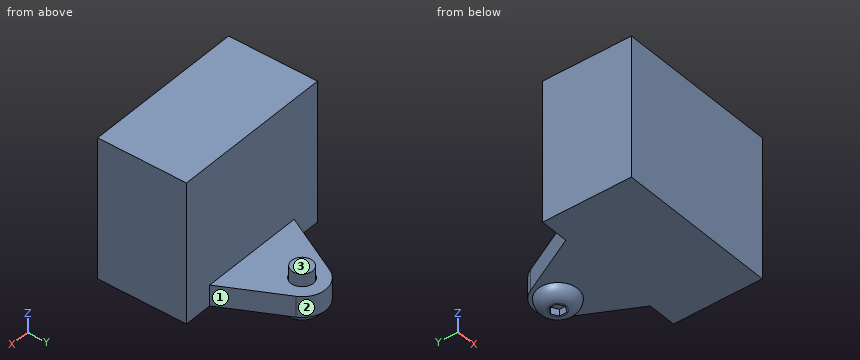
```python
from build123d import *

# Parameters (mm, degrees)
BOSS_EXTRUDE1_DEPTH = 4
SKETCH2_W           = 31
SKETCH2_H           = 17
BOSS_EXTRUDE2_DEPTH = 27
SKETCH4_R           = 2.15
CUT_EXTRUDE1_DEPTH  = 39.429285708
CUT_EXTRUDE2_DEPTH  = 1.3


with BuildPart() as part:
    # Sketch1 → Boss-Extrude1 (new body)
    with BuildSketch(Plane.XY.offset(-4)):
        with BuildLine():
            Line((-10, -9.6), (10, -9.6))
            Line((10, -9.6), (4.001428187, 2.058779362))
            ThreePointArc((4.001428187, 2.058779362), (0, 4.5), (-4.001428187, 2.058779362))
            Line((-4.001428187, 2.058779362), (-10, -9.6))
        make_face()
    extrude(amount=BOSS_EXTRUDE1_DEPTH)

    # Sketch2 → Boss-Extrude2 (add)
    with BuildSketch(Plane.XY.offset(-4)):
        with Locations((0, -18.1)):
            Rectangle(SKETCH2_W, SKETCH2_H)
    extrude(amount=BOSS_EXTRUDE2_DEPTH)

    # Sketch4 → Cut-Extrude1 (cut, through all)
    with BuildSketch(Plane.XY):
        Circle(SKETCH4_R)
    extrude(amount=-CUT_EXTRUDE1_DEPTH, mode=Mode.SUBTRACT)

    # Sketch5 → Revolve1 (revolve)
    with BuildSketch(Plane(origin=(0, 0, 0), x_dir=(0, 0, -1), z_dir=(1, 0, 0)), mode=Mode.PRIVATE) as revolve1_sk:
        with BuildLine():
            Line((-2.3, 0), (6.2, 0))
            Line((6.2, 0), (6.2, 1.6))
            ThreePointArc((6.2, 1.6), (5.555634919, 3.155634919), (4, 3.8))
            Line((4, 3.8), (4, 2))
            Line((4, 2), (-2.3, 2))
            Line((-2.3, 2), (-2.3, 0))
        make_face()
    revolve(revolve1_sk.sketch.rotate(Axis((0, 0, 2.3), (0, 0, -1)), 90), axis=Axis((0, 0, 2.3), (0, 0, -1)))

    # Sketch6 → Cut-Extrude2 (cut)
    with BuildSketch(Plane.XY.offset(-6.2)):
        Polygon((0, 1.443375673), (-1.25, 0.721687836), (-1.25, -0.721687836), (0, -1.443375673), (1.25, -0.721687836), (1.25, 0.721687836), align=None)
    extrude(amount=CUT_EXTRUDE2_DEPTH, mode=Mode.SUBTRACT)


solid = part.part
```
Work out the finished part from the listing and answer in its coordinate system (mm). Face numbers are marked on the shaded views. Give positions to 0.01 mm unless a question says otherwise; leave off trailing zeros. Order: outer loops, then holes, each group sorted by start corner. A loop starts at its lowest first (then second) coordinate and runs counter-clockwise, first axis right, second up. Notation, with made-up numbers: (42, -7.75) -> (72, -7.75) arc R24 cw to (72, 5.25) -> close; hole circle Ø3 at (51.25, 47). An arc over 180 degrees is marked (long way). Answer as CSV lines item,"result". Start each with the question number.
(1) Section B-B, the plane z = 9 is taken. Write down the section's boundary in (x, y), plus the area to 3 significant figures.
(2) Section C-C, the plane x = -5 is taken. Write down the section's boundary in (y, z).
(3) Section D-D, the plane y = -12.5 is taken. Write down the section's boundary in (x, z).
(4) Section A-A, the plane z = -0.75 is taken. Write down the section's boundary in (x, y), plus the area to 3 significant figures.
(5) Each of these flat-tipped pins is pushed along its axis until it touches: pin 1 Ø2 at (x, y) = (-10.5, -16) entering from -Z; pin 2 Ø1.5 at (x, z) = (2, 13) entering from +Y; pin 3 Ø1.2 at (x, y) = (0.5, 0) entering from -Z; pin 4 Ø1 at (y, z) = (-7.5, 3) entering from +X. Where does it stop, or does it pass through?
(6) For a pull along X with two mould halves and no side action, classify the marked faces 1, 2 and 3 as released by +X, released by -X, zero draft, split by the parting line, or undercut.
(7) Consider line 1 along Y through (x, z) = (11.5, 17.5); line 2 along Z through (x, y) = (-7, -18); line 3 along X through (y, z) = (3, -3.25). Determine where each line is inside the solid, lowest interval first.
Entries:
1,outline,"(-15.5, -26.6) -> (15.5, -26.6) -> (15.5, -9.6) -> (-15.5, -9.6) -> close"
1,area,"527 mm²"
2,outline,"(-26.6, -4) -> (0.12, -4) -> (0.12, 0) -> (-9.6, 0) -> (-9.6, 23) -> (-26.6, 23) -> close"
3,outline,"(-15.5, -4) -> (15.5, -4) -> (15.5, 23) -> (-15.5, 23) -> close"
4,outline,"(-15.5, -26.6) -> (15.5, -26.6) -> (15.5, -9.6) -> (10, -9.6) -> (4, 2.06) arc R4.5 ccw to (-4, 2.06) -> (-10, -9.6) -> (-15.5, -9.6) -> close; circle Ø4 at (0, 0); hole circle Ø4.3 at (0, 0)"
4,area,"702 mm²"
5,pin 1,"z = -4"
5,pin 2,"y = -9.6"
5,pin 3,"z = -4.9"
5,pin 4,"through"
6,face 1,"released by +X"
6,face 2,"split by the parting line"
6,face 3,"zero draft"
7,line 1,"-26.6 to -9.6"
7,line 2,"-4 to 23"
7,line 3,"-3.35 to 3.35"
